Model file for the job. Use its own axes, mm. Face numbers are marked on the shaded views. A direction names the side the tool comes from. Round coordinates to 2 decimals unless told otherwise and drop trailing zeros. Write each loop counter-clockwise with the first axis right and the second up, starting at its lowest first coordinate (ties: lowest second). Pieces come first, ordered by that corner, then holes.
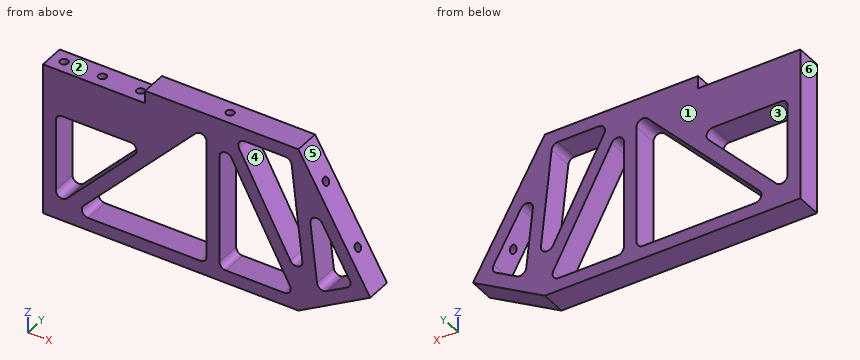
Autodesk Inventor part; units mm, degrees
ref_plane "YZ Plane" through (0, 0, 0) normal (1, 0, 0) x (0, 1, 0)
ref_plane "XZ Plane" through (0, 0, 0) normal (0, 1, 0) x (-1, 0, 0)
ref_plane "XY Plane" through (0, 0, 0) normal (0, 0, 1) x (1, 0, 0)
sketch "Sketch1" plane through (0, 0, 0) normal (0, 0, 1) x (1, 0, 0)
  line L0 (0, 0) -> (50.8, 0)
  line L1 (50.8, 0) -> (50.8, 12.7)
  line L2 (50.8, 12.7) -> (0, 12.7)
  line L3 (0, 12.7) -> (0, 0)
  dimension "d0" = 50.8
  dimension "d1" = 12.7
extrude "Extrusion1" add sketch "Sketch1" along normal blind 76.2
sketch "Sketch2" plane through (0, 0, 76.2) normal (0, 0, 1) x (1, 0, 0)
  line L0 (50.8, 12.7) -> (0, 12.7) construction
  line L1 (50.8, 0) -> (50.8, 12.7) construction
  line L2 (0, 12.7) -> (50.8, 12.7) construction
  line L3 (50.8, 12.7) -> (50.8, 6.35) construction
  line L4 (50.8, 6.35) -> (0, 6.35) construction
  line L5 (0, 6.35) -> (0, 12.7) construction
  point P0 (0, 0)
  point P1 (25.4, 6.35)
  point P2 (6.35, 6.35)
  point P3 (44.45, 6.35)
  dimension "d4" = 6.35
  dimension "d5" = 19.05
  dimension "d6" = 19.05
hole "Hole1" at (25.4, 6.35, 76.2) at (6.35, 6.35, 76.2) at (44.45, 6.35, 76.2) direction (0, 0, -1) diameter 3.9624 depth 16.51
sketch "Sketch3" plane through (50.8, 0, 0) normal (1, 0, 0) x (0, 0, -1)
  line L0 (0, 0) -> (-76.2, 0)
  line L1 (-76.2, 0) -> (-76.2, 12.7)
  line L2 (0, 0) -> (-76.2, 0)
  line L3 (-76.2, 0) -> (-76.2, 12.7)
  line L4 (-76.2, 12.7) -> (0, 12.7)
  line L5 (0, 12.7) -> (0, 0)
extrude "Extrusion2" add sketch "Sketch3" along normal blind 76.2
sketch "Sketch4" plane through (0, 0, 76.2) normal (0, 0, 1) x (1, 0, 0)
  line L0 (0, 12.7) -> (127, 12.7)
  line L1 (0, 0) -> (127, 0)
  line L2 (127, 12.7) -> (50.8, 12.7)
  line L3 (50.8, 12.7) -> (50.8, 0)
  line L4 (50.8, 0) -> (127, 0)
  line L5 (127, 0) -> (127, 12.7)
  dimension "d16" = 76.2
extrude "Extrusion3" add sketch "Sketch4" along normal blind 6.35
sketch "Sketch5" plane through (0, 0, 0) normal (0, -1, 0) x (1, 0, 0)
  line L0 (127, 0) -> (162.7452, 20.6375)
  line L1 (127, 0) -> (168.275, 0) construction
  line L2 (127, 0) -> (127, 82.55)
  line L3 (162.7452, 20.6375) -> (127, 82.55)
  line L4 (127, 82.55) -> (127, 0)
  point P0 (0, 0)
  dimension "d19" = 41.275
  dimension "d20" = 30
extrude "Extrusion4" add sketch "Sketch5" against normal up to surface (12.7 mm away)
sketch "Sketch6" plane through (0, 0, 76.2) normal (0, 1, 0) x (1, 0, 0)
  line L0 (4.3688, 16.51) -> (8.3312, 16.51)
  line L1 (8.3312, 0) -> (4.3688, 0)
  line L2 (8.3312, 0) -> (4.3688, 0)
  line L3 (4.3688, 16.51) -> (8.3312, 16.51)
  line L4 (0, 76.2) -> (0, 0)
  line L5 (0, 16.51) -> (50.8, 16.51)
  line L6 (50.8, 0) -> (50.8, -6.35)
  line L7 (50.8, 16.51) -> (50.8, 0)
  line L8 (0, 76.2) -> (127, 76.2)
  line L9 (6.35, 22.86) -> (6.35, 69.85)
  line L10 (6.35, 69.85) -> (50.8, 22.86)
  line L11 (50.8, 22.86) -> (6.35, 22.86)
  line L12 (57.15, 16.1471) -> (57.15, 0)
  line L13 (57.15, 0) -> (72.4243, 0)
  line L14 (72.4243, 0) -> (57.15, 16.1471)
  line L15 (127, -6.35) -> (50.8, -6.35)
  line L16 (6.35, 69.85) -> (10.9631, 74.2137) construction
  line L17 (10.9631, 74.2137) -> (15.0909, 69.85) construction
  line L18 (15.0909, 69.85) -> (81.4011, -0.2494)
  line L19 (81.4011, -0.2494) -> (81.4011, 69.85)
  line L20 (81.4011, 69.85) -> (15.0909, 69.85)
  line L21 (127, 76.2) -> (162.7452, 55.5625)
  line L22 (72.4243, 0) -> (77.0374, 4.3637) construction
  line L23 (77.0374, 4.3637) -> (81.4011, -0.2494) construction
  line L24 (87.7511, 0) -> (87.7511, 69.85)
  line L25 (87.7511, 69.85) -> (125.2985, 69.85)
  line L26 (125.2985, 69.85) -> (87.7511, 0)
  line L27 (130.8003, 66.6735) -> (94.9604, 0)
  line L28 (94.9604, 0) -> (123.3338, 0)
  line L29 (123.3338, 0) -> (130.8003, 66.6735)
  line L30 (162.7452, 55.5625) -> (127, -6.35)
  line L31 (136.802, 63.2085) -> (154.0709, 53.2382)
  line L32 (154.0709, 53.2382) -> (131.2611, 13.7305)
  line L33 (131.2611, 13.7305) -> (136.802, 63.2085)
  point P0 (6.35, 16.51)
  point P1 (57.15, 8.0736)
  point P2 (145.4365, 58.2234)
  dimension "d23" = 50.8
  dimension "d24" = 6.35
  dimension "d25" = 6.35
  dimension "d26" = 6.35
  dimension "d27" = 6.35
  dimension "d28" = 0
  dimension "d29" = 6.35
  dimension "d30" = 6.35
  dimension "d31" = 6.35
  dimension "d33" = 6.35
  dimension "d34" = 6.35
  dimension "d39" = 6.35
  dimension "d40" = 6.35
  dimension "d41" = 6.35
  dimension "d42" = 6.35
  dimension "d43" = 6.35
  dimension "d44" = 6.35
  dimension "d45" = 6.35
  dimension "d46" = 6.35
  dimension "d47" = 6.35
  dimension "d48" = 6.35
  dimension "d49" = 6.35
  dimension "d50" = 6.35
  dimension "d51" = 6.35
extrude "Extrusion5" cut sketch "Sketch6" along normal through all contours L9 L10 L11 | L20 L19 L18 | L24 L25 L26 | L29 L28 L27 | L31 L32 L33
fillet "Fillet1" radius 3.175 15 edges at (130.8003, 6.35, 9.5265) (136.802, 6.35, 12.9915) (154.0709, 6.35, 22.9618) (131.2611, 6.35, 62.4695) (94.9604, 6.35, 76.2) (123.3338, 6.35, 76.2) (125.2985, 6.35, 6.35) (87.7511, 6.35, 6.35) (87.7511, 6.35, 76.2) (81.4011, 6.35, 76.4494) (81.4011, 6.35, 6.35) (15.0909, 6.35, 6.35) (6.35, 6.35, 53.34) (50.8, 6.35, 53.34) (6.35, 6.35, 6.35)
sketch "Sketch7" plane through (0, 0, 82.55) normal (0, 0, 1) x (1, 0, 0)
  line L0 (127, 0) -> (127, 12.7) construction
  line L1 (127, 6.35) -> (50.8, 6.35) construction
  line L2 (50.8, 12.7) -> (50.8, 0) construction
  point P0 (0, 0)
  point P1 (88.9, 6.35)
hole "Hole2" at (88.9, 6.35, 82.55) direction (0, 0, -1) diameter 3.9624 depth 8.89
sketch "Sketch8" plane through (127, 0, 82.55) normal (0.8660254, 0, 0.5) x (0.5, 0, -0.8660254)
  line L0 (0, 0) -> (0, 12.7) construction
  line L1 (71.4904, 0) -> (71.4904, 12.7) construction
  line L2 (61.9654, 12.7) -> (34.7119, 12.7) construction
  point P0 (7.9904, 0)
  point P1 (19.05, 6.35)
  point P2 (50.8, 6.35)
  dimension "d69" = 19.05
  dimension "d70" = 31.75
hole "Hole3" at (136.525, 6.35, 66.0522) at (152.4, 6.35, 38.5559) direction (-0.8660254, 0, -0.5) diameter 3.9624 depth 8.89
sketch "Sketch9" plane through (0, 0, 0) normal (-1, 0, 0) x (0, 0, 1)
  line L0 (0, 12.7) -> (0, 0) construction
  line L1 (0, 6.35) -> (76.2, 6.35) construction
  point P0 (19.05, 6.35)
  point P1 (44.45, 6.35)
  point P2 (31.75, 6.35)
  dimension "d71" = 25.4
  dimension "d72" = 19.05
  dimension "d73" = 12.7
hole "Hole4" [suppressed]
chamfer "Chamfer1" [suppressed]
sketch "Sketch10" plane through (0, 0, 0) normal (0, -1, 0) x (1, 0, 0)
  line L0 (78.2261, 6.35) -> (22.4648, 6.35) construction
  line L1 (78.2261, 6.35) -> (81.4011, 6.35) construction
  arc A0 (78.2261, 6.35) -> (81.4011, 9.525) centre (78.2261, 9.525) ccw construction
  line L2 (81.4011, 6.35) -> (81.4011, 9.525) construction
  point P0 (0, 0)
  dimension "d84" = 3.175
sketch "Sketch11" plane through (0, 12.7, 76.2) normal (0, 1, 0) x (1, 0, 0)
  line L0 (78.2261, 69.85) -> (81.4011, 69.85) construction
  line L1 (81.4011, 69.85) -> (81.4011, 66.675) construction
  point P0 (0, 76.2)
properties part number "Third Baseplate"
1) Pull direction Z, two halves, no side cores. Call the marked faces 4, 5 and 6: released by +Z, released by -Z, zero draft, split by the parting line, or undercut.
2) Which spindle directions (+Z, -Z, +X, -X, +Y, -Y) get a long thin tool onto all of the face, cutting with end or side? Do the marked faces 1, 2 and 3. Say none if no direction does.
3) Cut at A-A on x = 16. List the corners of the cut face in (y, z), and give its area (3 significant figures).
4) Cut at C-C on x = 60. List the corners of the cut face in (y, z), and give its area (3 significant figures).
5) Wall check: probe 1 along Z at (x, y) = (33, 9.5); probe 2 along X at (y, z) = (8.5, 34); probe 3 along X at (y, z) = (3.5, 9.5). Give the ranges that are in metal, low to high.
6) Cut at B-B on x = 116. List the corners of the cut face in (y, z), and give its area (3 significant figures).
7) Flat gauge pins, fed straight in: pin 1 Ø1 at (x, y) = (133.5, 9.5) entering from +Z; pin 2 Ø2.5 at (x, y) = (88.9, 6.35) entering from +Z; pin 3 Ø1.2 at (x, y) = (26, 7) entering from +Z. Where does each tip first touch, or does it go through?
Result sheet:
1. face 4: undercut
1. face 5: released by +Z
1. face 6: zero draft
2. face 1: +Z, -Z, +X, -X, +Y
2. face 2: +Z, -X, +Y, -Y
2. face 3: +Y, -Y
3. outline: (0, 0) - (12.7, 0) - (12.7, 16.55) - (0, 16.55) - close; (0, 53.34) - (12.7, 53.34) - (12.7, 76.2) - (0, 76.2) - close
3. area: 501 mm2
4. outline: (0, 0) - (12.7, 0) - (12.7, 6.35) - (0, 6.35) - close; (0, 53.83) - (12.7, 53.83) - (12.7, 82.55) - (0, 82.55) - close
4. area: 445 mm2
5. probe 1: z = 0 to 6.35, 25.28 to 34.52, 53.34 to 76.2
5. probe 2: x = 0 to 6.35, 32.51 to 41.25, 81.4 to 87.75, 110.44 to 117.64, 128.06 to 134.45, 147.7 to 155.03
5. probe 3: x = 0 to 19.29, 81.4 to 87.75, 123.16 to 143.45
6. outline: (0, 0) - (12.7, 0) - (12.7, 6.35) - (0, 6.35) - close; (0, 23.65) - (12.7, 23.65) - (12.7, 37.06) - (0, 37.06) - close; (0, 76.2) - (12.7, 76.2) - (12.7, 82.55) - (0, 82.55) - close
6. area: 332 mm2
7. pin 1: stops at z = 72.16
7. pin 2: stops at z = 73.66
7. pin 3: stops at z = 59.69
